Part model, mm, in its own coordinate system. A direction names the side the tool comes from. Round coordinates to 2 decimals unless told otherwise and drop trailing zeros. Write each loop counter-clockwise with the first axis right and the second up, starting at its lowest first coordinate (ties: lowest second). Pieces come first, ordered by that corner, then holes. Notation, with made-up numbers: (62.5, -23.5) -> (109.5, -23.5) arc R33 ccw to (109.5, 14.5) -> close; hole circle Ø1 at (62, 13.25). An arc over 180 degrees is marked (long way). Use CSV: the item, a comma, the result in double quotes. Start each with the question number.
(1) Two-plate mould, pull along X, no slides. Class faces 6 (the cylindrical face through (18, 4, 0)), 7 (the flat face through (4, 37, 0)), 8 (the flat face through (3.7, 3.66, -5.18)): released by +X, released by -X, zero draft, split by the parting line, or undercut.
(2) Probe line 1 (Y direction, x = 6, z = 0); line 2 (X direction, y = 8, z = 1.5). List the from-to ranges inside material, lowest first. Write a range as [from, to].
(3) Saw through at D-D (x = 17). Give the cut face in (y, z).
(4) Saw through at C-C (x = 21). Give the cut face in (y, z), plus the area to 3 significant figures.
(5) Saw through at A-A (y = 25). Give the cut face in (x, z), plus the area to 4 significant figures.
(6) Drop flat-ended pins along their axis: pin 1 (5 mm diameter, centred on x = 21, z = 0, fed in from +Y); pin 2 (2.5 mm diameter, centred on y = 20, z = 5.5, fed in from +X); pin 3 (2.5 mm diameter, centred on x = 24.5, z = 0.5, fed in from +Y); pin 4 (6 mm diameter, centred on y = 25.5, z = 0.5, fed in from +X). Give the stop position or say it passes through.
(7) Which spindle directions (+Z, -Z, +X, -X, +Y, -Y) get a long thin tool onto all of the face, cutting with end or side? Do faces 1 (the flat face through (1.5, 24, 6)), 2 (the flat face through (4, 12, -5)), 3 (the flat face through (4, 12, 5)), 4 (the flat face through (6, 24, 6)), 5 (the flat face through (1.5, 24, -6)). Say none if no direction does.
(8) Saw through at B-B (z = 0). Give the cut face in (x, y).
```python
from build123d import *

# Parameters (mm, degrees)
SKETCH_1_W                = 31
SKETCH_1_H                = 37
EXTRUDE_1_DEPTH           = 7.8
SKETCH_2_W                = 23.5
SKETCH_2_H                = 29.5
CUT_EXTRUDE_1_DEPTH       = 49.896216623
SKETCH_3_W                = 29.18115942
SKETCH_3_H                = 5.9
EXTRUDE_2_DEPTH           = 3.35
SKETCH_4_W                = 4.5
SKETCH_4_H                = 25
EXTRUDE_3_DEPTH           = 3.35
SKETCH_5_W                = 4.5
SKETCH_5_H                = 25
EXTRUDE_4_DEPTH           = 3.35
SKETCH_6_W                = 29.18115942
SKETCH_6_H                = 5.9
EXTRUDE_5_DEPTH           = 3.35
DRAFT_1_ANGLE             = 45
DRAFT_2_ANGLE             = 45
DRAFT_3_ANGLE             = 57.901072745
DRAFT_4_ANGLE             = 57.901072745
HOLE_WIZARD_6_0_6_1_D     = 6
HOLE_WIZARD_6_0_6_2_D     = 6
HOLE_WIZARD_6_0_6_2_DEPTH = 37
CHAMFER_1_SIZE            = 1


with BuildPart() as part:
    # 草图1 → 凸台-拉伸1 (new body)
    with BuildSketch(Plane.XY.offset(3.9)):
        with Locations((15.5, 18.5)):
            Rectangle(SKETCH_1_W, SKETCH_1_H)
    extrude(amount=-EXTRUDE_1_DEPTH)

    # 草图2 → 切除-拉伸1 (cut, through all)
    with BuildSketch(Plane(origin=(0, 0, -3.9), x_dir=(-1, 0, 0), z_dir=(0, 0, -1))):
        with Locations((-19.25, 22.25)):
            Rectangle(SKETCH_2_W, SKETCH_2_H)
    extrude(amount=-CUT_EXTRUDE_1_DEPTH, mode=Mode.SUBTRACT)

    # 草图3 → 凸台-拉伸2 (add)
    with BuildSketch(Plane.XY.offset(3.9)):
        with Locations((16.25, 3.05)):
            Rectangle(SKETCH_3_W, SKETCH_3_H)
    extrude(amount=EXTRUDE_2_DEPTH)

    # 草图4 → 凸台-拉伸3 (add)
    with BuildSketch(Plane.XY.offset(3.9)):
        with Locations((3.75, 24.5)):
            Rectangle(SKETCH_4_W, SKETCH_4_H)
    extrude(amount=EXTRUDE_3_DEPTH)

    # 草图5 → 凸台-拉伸4 (add)
    with BuildSketch(Plane(origin=(0, 0, -3.9), x_dir=(-1, 0, 0), z_dir=(0, 0, -1))):
        with Locations((-3.75, 24.5)):
            Rectangle(SKETCH_5_W, SKETCH_5_H)
    extrude(amount=EXTRUDE_4_DEPTH)

    # 草图6 → 凸台-拉伸5 (add)
    with BuildSketch(Plane(origin=(0, 0, -3.9), x_dir=(-1, 0, 0), z_dir=(0, 0, -1))):
        with Locations((-16.25, 3.05)):
            Rectangle(SKETCH_6_W, SKETCH_6_H)
    extrude(amount=EXTRUDE_5_DEPTH)

    # 拔模1
    draft_1_faces = [part.faces().sort_by_distance(p)[0] for p in [
        (16.25, 0.1, -5.575),
    ]]
    draft(draft_1_faces, Plane(origin=(0, 0, -3.9), x_dir=(-1, 0, 0), z_dir=(0, 0, -1)), DRAFT_1_ANGLE)

    # 拔模2
    draft_2_faces = [part.faces().sort_by_distance(p)[0] for p in [
        (16.25, 0.1, 5.575),
    ]]
    draft(draft_2_faces, Plane.XY.offset(3.9), DRAFT_2_ANGLE)

    # 拔模3
    draft_3_faces = [part.faces().sort_by_distance(p)[0] for p in [
        (30.84057971, 3.776824458, -5.353648915),
        (1.65942029, 3.776824458, -5.353648915),
    ]]
    draft(draft_3_faces, Plane(origin=(0, 0, -3.9), x_dir=(-1, 0, 0), z_dir=(0, 0, -1)), DRAFT_3_ANGLE)

    # 拔模4
    draft_4_faces = [part.faces().sort_by_distance(p)[0] for p in [
        (30.84057971, 3.776824458, 5.353648915),
        (1.65942029, 3.776824458, 5.353648915),
    ]]
    draft(draft_4_faces, Plane.XY.offset(3.9), DRAFT_4_ANGLE)

    # Ø6.0 (6) 直径孔1 (through all)
    with Locations(Plane(origin=(7.5, 0, 0), x_dir=(0, 0, -1), z_dir=(1, 0, 0))):
        with Locations((0, 25)):
            Hole(HOLE_WIZARD_6_0_6_1_D / 2)

    # Ø6.0 (6) 直径孔2
    with Locations(Plane(origin=(0, 0, 0), x_dir=(-1, 0, 0), z_dir=(0, -1, 0))):
        with Locations((-21, 0)):
            Hole(HOLE_WIZARD_6_0_6_2_D / 2, depth=HOLE_WIZARD_6_0_6_2_DEPTH)

    # 倒角1
    chamfer_1_edges = [part.edges().sort_by_distance(p)[0] for p in [
        (3.75, 12, 7.25),
        (3.75, 37, 7.25),
        (3.75, 12, -7.25),
        (3.75, 37, -7.25),
    ]]
    chamfer(chamfer_1_edges, length=CHAMFER_1_SIZE)


solid = part.part
```
Answers:
1,face 6,"undercut"
1,face 7,"zero draft"
1,face 8,"released by -X"
2,line 1,"y = [0, 22], [28, 37]"
2,line 2,"x = [0, 7.5]"
3,outline,"(0, -3.9) -> (0.1, -3.9) -> (3.45, -7.25) -> (6, -7.25) -> (6, -3.9) -> (7.5, -3.9) -> (7.5, 3.9) -> (6, 3.9) -> (6, 7.25) -> (3.45, 7.25) -> (0.1, 3.9) -> (0, 3.9) -> close"
4,outline,"(0, -3.9) -> (0.1, -3.9) -> (3.45, -7.25) -> (6, -7.25) -> (6, -3.9) -> (7.5, -3.9) -> (7.5, -3) -> (0, -3) -> close; (0, 3) -> (7.5, 3) -> (7.5, 3.9) -> (6, 3.9) -> (6, 7.25) -> (3.45, 7.25) -> (0.1, 3.9) -> (0, 3.9) -> close"
4,area,"41.8 mm²"
5,outline,"(0, -3.9) -> (1.5, -3.9) -> (1.5, -7.25) -> (6, -7.25) -> (6, -3.9) -> (7.5, -3.9) -> (7.5, -3) -> (0, -3) -> close; (0, 3) -> (7.5, 3) -> (7.5, 3.9) -> (6, 3.9) -> (6, 7.25) -> (1.5, 7.25) -> (1.5, 3.9) -> (0, 3.9) -> close"
5,area,"43.65 mm²"
6,pin 1,"passes through"
6,pin 2,"stops at x = 6"
6,pin 3,"stops at y = 7.5"
6,pin 4,"stops at x = 7.5"
7,face 1,"+Z, -X, +Y, -Y"
7,face 2,"-Z, +X, -X"
7,face 3,"+Z, +X, -X"
7,face 4,"+Z, +X, +Y"
7,face 5,"-Z, -X, +Y, -Y"
8,outline,"(0, 0) -> (18, 0) -> (18, 7.5) -> (7.5, 7.5) -> (7.5, 22) -> (0, 22) -> close; (0, 28) -> (7.5, 28) -> (7.5, 37) -> (0, 37) -> close; (24, 0) -> (31, 0) -> (31, 7.5) -> (24, 7.5) -> close"
